```python
from build123d import *

# Parameters (mm, degrees)
SKETCH1_R           = 3.175
BOSS_EXTRUDE1_DEPTH = 0.79375


with BuildPart() as part:
    # Sketch1 → Boss-Extrude1 (new, symmetric)
    with BuildSketch(Plane.YZ):
        with BuildLine():
            Line((-138.9, 0), (-138.9, -43.2))
            Line((-138.9, -43.2), (-152.4, -43.2))
            Line((-152.4, -43.2), (-152.4, -41.2))
            ThreePointArc((-152.4, -41.2), (-153.19375, -40.40625), (-153.9875, -41.2))
            Line((-153.9875, -41.2), (-153.9875, -107.2))
            Line((-153.9875, -107.2), (-155.9875, -107.2))
            Line((-155.9875, -107.2), (-160.4, -82.175468971))
            Line((-160.4, -82.175468971), (-160.4, -18.524531029))
            Line((-160.4, -18.524531029), (-155.9875, 6.5))
            Line((-155.9875, 6.5), (-145.4, 6.5))
            ThreePointArc((-145.4, 6.5), (-140.803805922, 4.596194078), (-138.9, 0))
        make_face()
        with Locations(Location((-145.4, 0, 0), (0, 0, 270))):
            Circle(SKETCH1_R, mode=Mode.SUBTRACT)
    extrude(amount=BOSS_EXTRUDE1_DEPTH, both=True)


solid = part.part
```
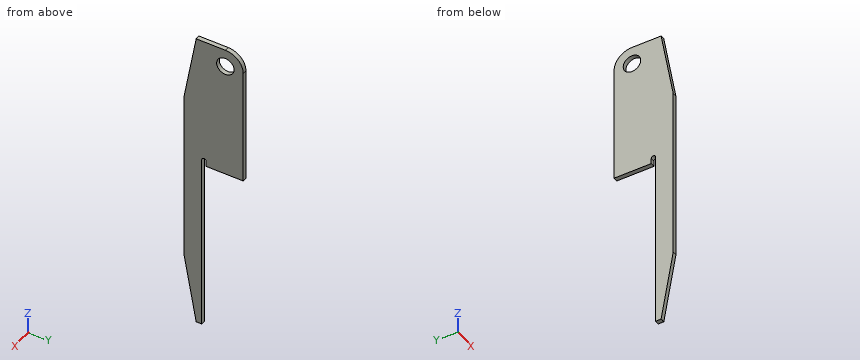
Check sheet for the modelled part. Datum: model origin and axes. Units: mm. Give positions to 0.01 mm unless a question says otherwise; leave off trailing zeros. Order: outer loops, then holes, each group sorted by start corner. A loop starts at its lowest first (then second) coordinate and runs counter-clockwise, first axis right, second up. Notation, with made-up numbers: (72, 7.25) -> (120, 7.25) arc R20 cw to (120, 38.25) -> close; hole circle Ø5 at (41, 87.5). An arc over 180 degrees is marked (long way). Use CSV: the item, a comma, the result in double quotes. Start each with the question number.
1) Sectioned sample at C-C, the plane z = -60.5. Record the boundary of the cut face in (x, y).
2) Go/stop test with flat-tipped pins: P1, Ø0.8, axis at x = -0.5, y = -142.5, coming from the -Z side; P2, Ø10, axis at y = -145, z = -48, coming from the -X side. Record where each tip stops, or that it passes through.
3) Sectioned sample at B-B, the plane y = -144.25. Record the boundary of the cut face in (x, z).
4) Material ranges on line 1 (Z direction, x = -0.35, y = -145.4) (3 decimals); line 2 (Y direction, x = -0.6, z = -41.5); line 3 (Y direction, x = 0.6, z = -67.5), recorded low to high. Write a range as from..to.
5) Sectioned sample at D-D, the plane z = -94. Record the boundary of the cut face in (x, y).
Recorded:
1,outline,"(-0.79, -160.4) -> (0.79, -160.4) -> (0.79, -153.99) -> (-0.79, -153.99) -> close"
2,P1,"z = -43.2"
2,P2,"x = -0.79"
3,outline,"(-0.79, -43.2) -> (0.79, -43.2) -> (0.79, -2.96) -> (-0.79, -2.96) -> close; (-0.79, 2.96) -> (0.79, 2.96) -> (0.79, 6.4) -> (-0.79, 6.4) -> close"
4,line 1,"-43.2..-3.175, 3.175..6.5"
4,line 2,"-160.4..-153.99, -152.4..-138.9"
4,line 3,"-160.4..-153.99"
5,outline,"(-0.79, -158.32) -> (0.79, -158.32) -> (0.79, -153.99) -> (-0.79, -153.99) -> close"
